```python
from build123d import *

# Parameters (mm, degrees)
BOSS_EXTRUDE1_DEPTH = 5.5


with BuildPart() as part:
    # Sketch1 → Boss-Extrude1 (new body)
    with BuildSketch(Plane.XY):
        Polygon((-264.257200354, -90.158072964), (-264.257200354, -95.658072964), (-230.257200354, -95.658072964), (-230.257200354, -90.158072964), (-195.597200354, -90.158072964), (-195.597200354, -95.658072964), (-161.597200354, -95.658072964), (-161.597200354, -90.158072964), (-126.917200354, -90.158072964), (-126.917200354, -95.658072964), (-92.917200354, -95.658072964), (-92.917200354, -90.158072964), (-58.257200354, -90.158072964), (-58.257200354, -95.658072964), (-24.257200354, -95.658072964), (-24.257200354, -90.158072964), (-24.257200354, 4.28308251), (-141.707906421, -51.738030582), (-144.075717453, -46.773811518), (64.743830776, 52.828003736), (-1.770133681, 192.277430168), (-254.494013299, 71.734323062), (-191.424137459, -60.49442102), (-205.726515812, -67.316305554), (-212.73562074, -52.621411895), (-222.803045061, -57.423326974), (-240.553810667, -20.208072964), (-264.257200354, -20.208072964), align=None)
        Polygon((-226.65672616, -81.398839397), (-231.134041567, -72.01195244), (-225.718529861, -69.428885859), (-221.241214454, -78.815772816), align=None, mode=Mode.SUBTRACT)
        Polygon((-214.729005488, -68.418450138), (-219.206320895, -59.031563181), (-214.151843303, -56.620701038), (-209.674527896, -66.007587996), align=None, mode=Mode.SUBTRACT)
        Polygon((-233.682985152, -52.731058098), (-229.205669745, -62.117945056), (-234.621181451, -64.701011637), (-239.098496858, -55.314124679), align=None, mode=Mode.SUBTRACT)
        Polygon((-241.647440443, -36.033230338), (-237.170125036, -45.420117295), (-242.585636742, -48.003183876), (-247.062952149, -38.616296919), align=None, mode=Mode.SUBTRACT)
        Polygon((-168.861811902, 101.721088208), (-166.321796431, 96.39583503), (-184.734536232, 87.613408655), (-187.274551703, 92.938661833), align=None, mode=Mode.SUBTRACT)
        Polygon((-60.55157778, 153.382419825), (-58.011562309, 148.057166647), (-76.42430211, 139.274740272), (-78.964317581, 144.59999345), align=None, mode=Mode.SUBTRACT)
    extrude(amount=BOSS_EXTRUDE1_DEPTH)


solid = part.part
```
The model under review builds one solid part; all positions refer to its coordinate system, in mm. A direction names the side the tool comes from. Round coordinates to 2 decimals unless told otherwise and drop trailing zeros. Order: outer loops, then holes, each group sorted by start corner. A loop starts at its lowest first (then second) coordinate and runs counter-clockwise, first axis right, second up. Notation, with made-up numbers: (-33.75, -27) - (1.25, -27) arc R8 cw to (1.25, -17) - close; hole circle Ø7 at (85.5, -0.5). An arc over 180 degrees is marked (long way). Answer in a Markdown table with one row per item.
(1) Machinability: for faces 1 (the face through (-102, 18, 5.5)), 2 (the face through (-41.13, 2.33, 2.71)), which of the approach directions +Z, -Z, +X, -X, +Y, -Y give a long, thin tool a straight path to every point of the face, cutting with its end or side? Answer none if there is none.
Result set:
| item | result |
|---|---|
| face 1 | +Z, +X, -X, +Y, -Y |
| face 2 | +Z, -Z |
(2) Take a section at B-B on z = 3.85. Count the separate pieces of the cut face and the enclosed holes in it, plus the area to 3 significant figures.
Result set:
| item | result |
|---|---|
| separate pieces | 1 |
| enclosed holes | 6 |
| area | 56,500 mm2 |
(3) Take a section at D-D on x = -18. Write out the cut boundary in (y, z), plus the area to 3 significant figures.
Result set:
| item | result |
|---|---|
| outline | (13.36, 0) - (184.54, 0) - (184.54, 5.5) - (13.36, 5.5) - close |
| area | 941 mm2 |
(4) Mouldability with a two-part tool opening along Y and no side actions: class faces 3 (the face through (-69.89, 148.93, 2.71)), 4 (the face through (-126.36, 132.85, 2.71)), 5 (the face through (-102, 18, 0)) as released by +Y, released by -Y, zero draft, split by the parting line, or undercut.
Result set:
| item | result |
|---|---|
| face 3 | undercut |
| face 4 | released by +Y |
| face 5 | zero draft |
(5) Clearance check with flat-ended pins moving along their axes: P1, Ø2, axis at y = 107.5, z = 2.5, coming from the -X side; P2, Ø3, axis at x = 25.5, z = 2, coming from the +Y side; P3, Ø3, axis at y = -57, z = 4, coming from the +X side; P4, Ø1.5, axis at x = -80.5, y = 125, coming from the -Z side. State where each tip first meets the part, or that it passes through.
Result set:
| item | result |
|---|---|
| P1 | stops at x = -181.61 |
| P2 | stops at y = 138.25 |
| P3 | stops at x = -24.26 |
| P4 | stops at z = 0 |
(6) Take a section at A-A on x = -135. Write out the cut boundary in (y, z), plus the area to 3 significant figures.
Result set:
| item | result |
|---|---|
| outline | (-90.16, 0) - (-48.54, 0) - (-48.54, 5.5) - (-90.16, 5.5) - close; (-42.44, 0) - (128.73, 0) - (128.73, 5.5) - (-42.44, 5.5) - close |
| area | 1,170 mm2 |
(7) For line 1 (X direction, y = -55, z = 5.2); line 2 (Y direction, x = -227.5, z = 0.45); line 3 (X direction, y = -21.5, z = 4.35), list the stretches that pass through material, from the lowest coordinate up. Write a range as from..to.
Result set:
| item | result |
|---|---|
| line 1 | x = -264.26..-238.44, -232.6..-223.96, -217.72..-211.6, -194.04..-24.26 |
| line 2 | y = -90.16..-79.63, -70.28..-47.58, 15.14..84.61 |
| line 3 | x = -264.26..-239.94, -210.02..-91.09, -78.31..-24.26 |
(8) Take a section at C-C on y = 32.5. Write out the cut boundary in (x, z), plus the area to 3 significant figures.
Result set:
| item | result |
|---|---|
| outline | (-235.78, 0) - (22.13, 0) - (22.13, 5.5) - (-235.78, 5.5) - close |
| area | 1,420 mm2 |
